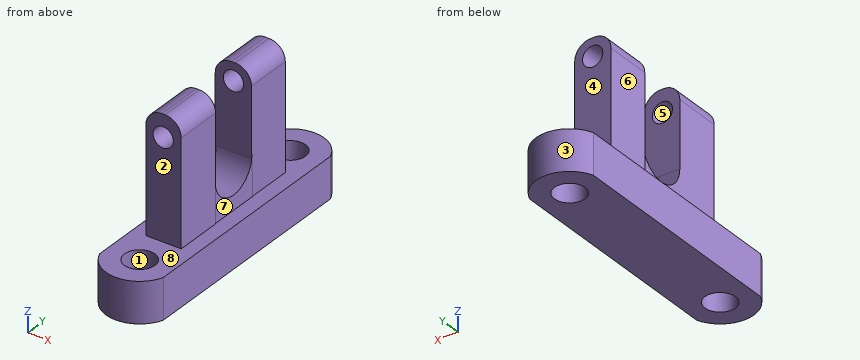
from build123d import *

# Parameters (mm, degrees)
F0_R      = 4.789486544
F1_DEPTH  = 12.7
F2_W      = 11.0857239924
F2_H      = 14.9416252971
F3_DEPTH  = 38.1
F5_D      = 6.35
F6_R      = 5.08
F8_W      = 11.3267181441
F8_H      = 14.700633008
F9_DEPTH  = 38.1
F11_D     = 6.35
F11_DEPTH = 25.4
F11_TIP   = 1.9077324654
F12_R     = 5.08
F14_DEPTH = 10.922


with BuildPart() as f1:
    # F0 (on Top) → F1 (new body)
    with BuildSketch(Plane.XY):
        with BuildLine():
            ThreePointArc((0, 32.4136912823), (-9.941002354, 39.4109395409), (-19.8820047081, 32.4136912823))
            Line((-19.8820047081, 32.4136912823), (-19.8820047081, -40.1254966855))
            ThreePointArc((-19.8820047081, -40.1254966855), (-9.941002354, -47.1227449441), (0, -40.1254966855))
            Line((0, -40.1254966855), (0, 32.4136912823))
        make_face()
        with Locations((-9.941002354, -36.5625214439)):
            Circle(F0_R, mode=Mode.SUBTRACT)
        with Locations((-9.941002354, 28.8507160407)):
            Circle(F0_R, mode=Mode.SUBTRACT)
    extrude(amount=F1_DEPTH)

    # F2 (on face) → F3 (join)
    with BuildSketch(Plane.XY.offset(12.7)):
        with Locations((-10.0012498442, -18.677033484)):
            Rectangle(F2_W, F2_H)
    extrude(amount=F3_DEPTH)

    # F5 (through all)
    with Locations(Plane.XZ.offset(26.1478461325)):
        with Locations((-10.0886579603, 43.8547693193)):
            Hole(F5_D / 2)

    # F6
    f6_edges = [f1.edges().sort_by_distance(p)[0] for p in [
        (-4.458388, -18.677033, 50.8),
        (-15.544112, -18.677033, 50.8),
    ]]
    fillet(f6_edges, radius=F6_R)

    # F8 (on face) → F9 (join)
    with BuildSketch(Plane.XY.offset(12.7)):
        with Locations((-10.3627410717, 12.0496989693)):
            Rectangle(F8_W, F8_H)
    extrude(amount=F9_DEPTH)

    # F11
    with Locations(Plane(origin=(0, 19.4000154734, 0), x_dir=(-1, 0, 0), z_dir=(0, 1, 0))):
        with Locations((10.3249410167, 45.2776290476)):
            Hole(F11_D / 2, depth=F11_DEPTH)
            with Locations((0, 0, -(F11_DEPTH + F11_TIP / 2))):  # 118° drill point
                Cone(0, F11_D / 2, F11_TIP, mode=Mode.SUBTRACT)

    # F12
    f12_edges = [f1.edges().sort_by_distance(p)[0] for p in [
        (-4.699382, 12.049699, 50.8),
        (-16.0261, 12.049699, 50.8),
    ]]
    fillet(f12_edges, radius=F12_R)

    # F13 (on face) → F14 (join)
    with BuildSketch(Plane(origin=(-15.5441118404, 0, 0), x_dir=(0, -1, 0), z_dir=(-1, 0, 0))):
        with BuildLine():
            Line((11.2062208354, 25.3779198974), (11.2062208354, 25.1054665343))
            ThreePointArc((11.2062208354, 25.1054665343), (11.2073811699, 25.2416932159), (11.2062208354, 25.3779198974))
        make_face()
        with BuildLine():
            ThreePointArc((11.2062208354, 25.1054665343), (3.0232009523, 17.2465905604), (-4.783663433, 25.4792459309))
            Line((-4.783663433, 25.4792459309), (-5.1880729605, 11.8706798134))
            Line((-5.1880729605, 11.8706798134), (11.2062208354, 12.7))
            Line((11.2062208354, 12.7), (11.2062208354, 25.1054665343))
        make_face()
    extrude(amount=-F14_DEPTH)


solid = f1.part
Can you work these out from the model? Positions are in its coordinate system, mm. Face numbers are marked on the shaded views. A direction names the side the tool comes from. Round coordinates to 2 decimals unless told otherwise and drop trailing zeros. Order: outer loops, then holes, each group sorted by start corner. A loop starts at its lowest first (then second) coordinate and runs counter-clockwise, first axis right, second up. Notation, with made-up numbers: M 5.25,69.25 L 44.25,69.25 A10 ccw 44.25,88.25 Z; hole C 27,-29 d7. An arc over 180 degrees is marked long. Use a Markdown table: item, result.
1) Imagine slicing it at C-C (y = 27.5). List the corners of the cut face in (x, z) for me, then the cut area to 3 significant figures.
Geometry says:
| item | result |
|---|---|
| outline | M -19.88,0 L -14.54,0 L -14.54,12.7 L -19.88,12.7 Z; M -5.35,0 L 0,0 L 0,12.7 L -5.35,12.7 Z |
| area | 136 mm² |
2) On a 3-axis mill with a long thin cutter (end or side, diameter ignored), from which of +Z, -Z, +X, -X, +Y, -Y can I reach the whole of each face in a straight line? I mean the marked faces 4, 5, 6, 7 and 8. Say none if no direction works.
Geometry says:
| item | result |
|---|---|
| face 4 | +Z, +X, -X, +Y |
| face 5 | -Y |
| face 6 | +Z, -X, +Y, -Y |
| face 7 | +Z, +X, +Y |
| face 8 | +Z |
3) Imagine slicing it at B-B (y = -17). List the corners of the cut face in (x, z) for me (3 decimals).
Geometry says:
| item | result |
|---|---|
| outline | M -19.882,0 L 0,0 L 0,12.7 L -4.458,12.7 L -4.458,45.72 A5.08 ccw -9.538,50.8 L -10.464,50.8 A5.08 ccw -15.544,45.72 L -15.544,12.7 L -19.882,12.7 Z; hole C -10.089,43.855 d6.35 |
4) Imagine slicing it at D-D (z = 8). List the corners of the cut face in (x, y) for me.
Geometry says:
| item | result |
|---|---|
| outline | M -19.88,-40.13 A10.56 ccw 0,-40.13 L 0,32.41 A10.56 ccw -19.88,32.41 Z; hole C -9.94,-36.56 d9.58; hole C -9.94,28.85 d9.58 |
5) If we mould it in two halves opening along Y, with no side actions, what happens to the marked faces 1, 2 and 3? For each: +Y half, -Y half, draft (parallel to the pull), parting line (faces both ways), or undercut.
Geometry says:
| item | result |
|---|---|
| face 1 | undercut |
| face 2 | -Y half |
| face 3 | +Y half |
6) I'm going to push flat-ended pins straight in: P1, Ø5.5, axis at x = -11, z = 38.5, coming from the +Y side; P2, Ø5.5, axis at x = -11, z = 32, coming from the -Y side; P3, Ø5, axis at x = -10.32, z = 45.28, coming from the +Y side. Where does each tip first touch, or does it pass through?
Geometry says:
| item | result |
|---|---|
| P1 | stops at y = 19.4 |
| P2 | stops at y = -26.15 |
| P3 | stops at y = -11.21 |
7) If I drill on line 1 along Y through (x, z) = (-11.5, 40.5); line 2 along Z through (x, y) = (-17.5, 9.5); line 3 along Y through (x, z) = (-8, 13), over which ranges is the centre line in solid material (lowest first)?
Geometry says:
| item | result |
|---|---|
| line 1 | y = -26.15 to -11.21, 4.7 to 19.4 |
| line 2 | z = 0 to 12.7 |
| line 3 | y = -26.15 to 19.4 |
8) Imagine slicing it at A-A (z = 32.5). List the corners of the cut face in (x, y) for me, then the cut area to 3 significant figures.
Geometry says:
| item | result |
|---|---|
| outline | M -16.03,4.7 L -4.7,4.7 L -4.7,19.4 L -16.03,19.4 Z; M -15.54,-26.15 L -4.46,-26.15 L -4.46,-11.21 L -15.54,-11.21 Z |
| area | 332 mm² |
